Can you work these out from the model? Positions are in its coordinate system, mm. Face numbers are marked on the shaded views. A direction names the side the tool comes from. Coordinates: 2 decimals unless noted, no trailing zeros. Loops run counter-clockwise (first coordinate to the right, second up) from the corner with the lowest first, then second, coordinate; pieces in that order, holes last.
```python
from build123d import *

# Parameters (mm, degrees)
F0_W     = 170
F0_H     = 100
F1_DEPTH = 1.5
F2_R     = 8.25
F2_W     = 13
F2_H     = 30
F2_R_2   = 2
F3_DEPTH = 25
F4_W     = 20
F4_H     = 13
F5_DEPTH = 3.5
F6_W     = 18.5
F6_H     = 13
F7_DEPTH = 1


# Not quite as in the source:
# - a pattern or mirror of a feature is missing from the dataset's text; its kind, count and spacing are read off the source's solid


with BuildPart() as f1:
    # F0 (on Front) → F1 (new body)
    with BuildSketch(Plane.XZ):
        Rectangle(F0_W, F0_H)
    extrude(amount=F1_DEPTH)

    # F2 (on face) → F3 (cut)
    with BuildSketch(Plane.XZ.offset(1.5)):
        with Locations((30.75, -34.75)):
            Circle(F2_R)
        with Locations((30.75, -8.25)):
            Circle(F2_R)
        with Locations((30.75, 18.25)):
            Circle(F2_R)
        with Locations((1, -10)):
            Rectangle(F2_W, F2_H)
        with Locations((-26, -35)):
            Circle(F2_R_2)
        with Locations((-26, 18)):
            Circle(F2_R_2)
    extrude(amount=-F3_DEPTH, mode=Mode.SUBTRACT)

    # F4 (on face) → F5 (join)
    with BuildSketch(Plane.YZ.offset(85)):
        with Locations((8.5, -43.5)):
            Rectangle(F4_W, F4_H)
    f5 = extrude(amount=F5_DEPTH)

    # F5_copies: F5 across plane
    add(f5.mirror(Plane(origin=(0, 0, 0), x_dir=(0, 0, -1), z_dir=(-1, 0, 0))))

    # F6 (on face) → F7 (cut)
    with BuildSketch(Plane(origin=(85, 0, 0), x_dir=(0, -1, 0), z_dir=(-1, 0, 0))):
        with Locations((-9.25, -43.5)):
            Rectangle(F6_W, F6_H)
    f7 = extrude(amount=-F7_DEPTH, mode=Mode.SUBTRACT)

    # F7_copies: F7 across plane
    add(f7.mirror(Plane(origin=(0, 0, 0), x_dir=(0, 0, -1), z_dir=(-1, 0, 0))), mode=Mode.SUBTRACT)


solid = f1.part
```
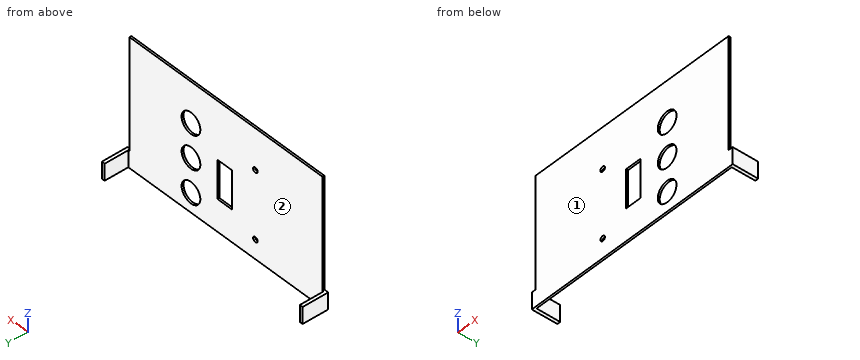
(1) I want a section at B-B on z = -8.25. Write out the boundary of the cut face in (x, y), then the cut area to 3 significant figures.
Check values:
outline: (-85, -1.5) - (-5.5, -1.5) - (-5.5, 0) - (-85, 0) - close; (7.5, -1.5) - (22.5, -1.5) - (22.5, 0) - (7.5, 0) - close; (39, -1.5) - (85, -1.5) - (85, 0) - (39, 0) - close
area: 211 mm2
(2) I want a section at C-C on x = 30.75. Write out the boundary of the cut face in (y, z).
Check values:
outline: (-1.5, -50) - (0, -50) - (0, -43) - (-1.5, -43) - close; (-1.5, -26.5) - (0, -26.5) - (0, -16.5) - (-1.5, -16.5) - close; (-1.5, 0) - (0, 0) - (0, 10) - (-1.5, 10) - close; (-1.5, 26.5) - (0, 26.5) - (0, 50) - (-1.5, 50) - close
(3) I'm going to push flat-ended pins straight in: pin 1 (8 mm diameter, centred on y = 5.5, z = 36.5, fed in from -X); pin 2 (0.8 mm diameter, centred on y = -0.5, z = -16, fed in from +X); pin 3 (1.8 mm diameter, centred on x = 87.5, y = 8.5, fed in from +Z); pin 4 (1.2 mm diameter, centred on y = -1, z = 18.5, fed in from -X). Where does each tip first touch, or does it pass through?
Check values:
pin 1: passes through
pin 2: stops at x = 85
pin 3: stops at z = -37
pin 4: stops at x = -85
(4) Which directions (+Z, -Z, +X, -X, +Y, -Y) give clear straight access to the entire face, cutting with the end or side of a thin tool? Please do the marked faces 1 and 2.
Check values:
face 1: +Z, -Z, +X, -X, -Y
face 2: +Z, -Z, +Y
(5) I want a section at A-A on x = 4.5. Write out the boundary of the cut face in (y, z).
Check values:
outline: (-1.5, -50) - (0, -50) - (0, -25) - (-1.5, -25) - close; (-1.5, 5) - (0, 5) - (0, 50) - (-1.5, 50) - close
(6) I want a section at D-D on y = 15.25. Write out the boundary of the cut face in (x, z).
Check values:
outline: (-88.5, -50) - (-86, -50) - (-86, -37) - (-88.5, -37) - close; (86, -50) - (88.5, -50) - (88.5, -37) - (86, -37) - close
(7) If I drill on probe 1 along Z at (x, y) = (30.75, -0.8); probe 2 along Z at (x, y) = (-26, -0.8); probe 3 along X at (y, z) = (7.25, -39), over which ranges is the centre line in solid material (lowest first)?
Check values:
probe 1: z = -50 to -43, -26.5 to -16.5, 0 to 10, 26.5 to 50
probe 2: z = -50 to -37, -33 to 16, 20 to 50
probe 3: x = -88.5 to -86, 86 to 88.5
